For this review, take the finished solid that the model builds, in its own axes (mm). Give positions to 0.01 mm unless a question says otherwise; leave off trailing zeros. Order: outer loops, then holes, each group sorted by start corner. A loop starts at its lowest first (then second) coordinate and runs counter-clockwise, first axis right, second up. Notation, with made-up numbers: M 38.25,78 L 95.25,78 A23 ccw 95.25,111 Z; hole C 35.25,38.5 d6. An arc over 180 degrees is marked long. Answer as CSV lines item,"result". Start each with the question number.
1. For line 1 along Z through (x, y) = (2.1, 5); line 2 along Z through (x, y) = (2.05, 25); line 3 along Y through (x, z) = (2.5, 20), list the stretches that pass through material, from the lowest coordinate up.
2. We need section B-B, the plane y = 5. Give the boundary of the cut face in (x, z), and give its area (3 significant figures).
3. Mouldability with a two-part tool opening along Y and no side actions: class faces 1 (the cylindrical face through (1.521, 58.84, 39.773)), 2 (the cylindrical face through (1.479, 3.526, 10.648)), 3 (the flat face through (1, 0, 20)) as pulls with the +Y half, pulls with the -Y half, needs draft (parallel to the pull), parting line crosses it, or undercut.
4. We need section C-C, the plane z = 12. Give the boundary of the cut face in (x, y), and give its area (3 significant figures).
5. We need section A-A, the plane y = 25. Give the boundary of the cut face in (x, z).
6. We need section D-D, the plane x = 0.55. Give the boundary of the cut face in (y, z).
Autodesk Inventor part; units mm, degrees
ref_plane "YZ Plane" through (0, 0, 0) normal (1, 0, 0) x (0, 1, 0)
ref_plane "XZ Plane" through (0, 0, 0) normal (0, 1, 0) x (-1, 0, 0)
ref_plane "XY Plane" through (0, 0, 0) normal (0, 0, 1) x (1, 0, 0)
sketch "Sketch1" plane through (0, 0, 0) normal (1, 0, 0) x (0, 1, 0)
  line L0 (0, 0) -> (0, 40)
  line L1 (0, 40) -> (82, 40) construction
  line L2 (82, 40) -> (43, 0) construction
  line L3 (43, 0) -> (0, 0)
  line L4 (85.0695, 14.499) -> (70.933, 0)
  line L5 (70.933, 0) -> (43, 0)
  line L6 (85.0695, 14.499) -> (70.7495, 28.461)
  circle A0 centre (75.1171, 18.616) radius 2
  circle A1 centre (63.9475, 7.16) radius 2
  line L7 (77.9095, 21.48) -> (56.9665, 0) construction
  circle A2 centre (25, 32) radius 2
  circle A3 centre (5, 32) radius 2
  circle A4 centre (5, 12) radius 2
  line L8 (25, 32) -> (5, 32) construction
  line L9 (5, 32) -> (5, 12) construction
  line L10 (70.7495, 28.461) -> (58.9146, 40)
  line L11 (0, 40) -> (58.9146, 40)
  dimension "d0" = 43
  dimension "d1" = 39
  dimension "d2" = 40
  dimension "d4" = 4
  dimension "d5" = 16
  dimension "d6" = 4
  dimension "d7" = 4
  dimension "d8" = 20
  dimension "d9" = 20
  dimension "d10" = 8
  dimension "d11" = 5
  dimension "d16" = 20
  dimension "d17" = 10
extrude "Extrusion1" add sketch "Sketch1" along normal blind 3
fillet "Fillet1" radius 3 4 edges at (1.5, 58.9146, 40) (1.5, 70.933, 0) (1.5, 0, 40) (1.5, 0, 0)
fillet "Fillet2" radius 8 1 edges at (1.5, 85.0695, 14.499)
properties part number "Arm_Servo_Holder"
Result set:
1,line 1,"0 to 10, 14 to 30, 34 to 40"
1,line 2,"0 to 30, 34 to 40"
1,line 3,"0 to 73.67, 76.56 to 79.43"
2,outline,"M 0,0 L 3,0 L 3,10 L 0,10 Z; M 0,14 L 3,14 L 3,30 L 0,30 Z; M 0,34 L 3,34 L 3,40 L 0,40 Z"
2,area,"96.0 mm2"
3,face 1,"pulls with the +Y half"
3,face 2,"undercut"
3,face 3,"pulls with the -Y half"
4,outline,"M 0,0 L 3,0 L 3,3 L 0,3 Z; M 0,7 L 3,7 L 3,81.4 L 0,81.4 Z"
4,area,"232 mm2"
5,outline,"M 0,0 L 3,0 L 3,30 L 0,30 Z; M 0,34 L 3,34 L 3,40 L 0,40 Z"
6,outline,"M 0,3 A3 ccw 3,0 L 69.67,0 A3 ccw 71.82,0.91 L 79.48,8.77 A8 ccw 79.34,20.08 L 70.75,28.46 L 59.79,39.15 A3 ccw 57.69,40 L 3,40 A3 ccw 0,37 Z; hole C 5,12 d4; hole C 5,32 d4; hole C 25,32 d4; hole C 63.95,7.16 d4; hole C 75.12,18.62 d4"
